from build123d import *

# Parameters (mm, degrees)
S2D0001_W           = 69.85
S2D0001_H           = 100.076
BOSS_EXTRUDE1_DEPTH = 3.175
FILLET1_R           = 3.175
S2D0002_R           = 1.27
CUT_EXTRUDE1_DEPTH  = 3.4925
BOSS_EXTRUDE2_DEPTH = 1.27
FILLET2_R           = 2.54
FILLET3_R           = 1.016
BOSS_EXTRUDE3_DEPTH = 6.35
S2D0005_W           = 5.08
S2D0005_H           = 6.35
BOSS_EXTRUDE4_DEPTH = 69.85
BOSS_EXTRUDE5_DEPTH = 0.889
BOSS_EXTRUDE6_DEPTH = 6.35


with BuildPart() as part:
    # S2D0001 → Boss-Extrude1 (new body)
    with BuildSketch(Plane(origin=(0, 0, 0), x_dir=(1, 0, 0), z_dir=(0, 1, 0))):
        with Locations((34.925, 50.038)):
            Rectangle(S2D0001_W, S2D0001_H)
    extrude(amount=-BOSS_EXTRUDE1_DEPTH)

    # Fillet1
    fillet1_edges = [part.edges().sort_by_distance(p)[0] for p in [
        (69.85, -1.5875, 0),
    ]]
    fillet(fillet1_edges, radius=FILLET1_R)

    # S2D0002 → Cut-Extrude1 (cut)
    with BuildSketch(Plane(origin=(0, 0, 0), x_dir=(1, 0, 0), z_dir=(0, 1, 0))):
        with Locations((3.175, 96.901)):
            Circle(S2D0002_R)
        with Locations((66.675, 96.901)):
            Circle(S2D0002_R)
        with Locations((3.175, 50.038)):
            Circle(S2D0002_R)
        with Locations((66.675, 50.038)):
            Circle(S2D0002_R)
        with Locations((3.175, 3.175)):
            Circle(S2D0002_R)
        with Locations((66.675, 3.175)):
            Circle(S2D0002_R)
    extrude(amount=-CUT_EXTRUDE1_DEPTH, mode=Mode.SUBTRACT)

    # Sketch3 → Boss-Extrude2 (add)
    with BuildSketch(Plane(origin=(0, 0, 0), x_dir=(-1, 0, 0), z_dir=(0, 1, 0))):
        with BuildLine():
            Line((-9.493170226, -96.266), (-59.69, -96.266))
            Line((-59.69, -96.266), (-66.04, -89.916))
            Line((-66.04, -89.916), (-66.04, -56.356170226))
            ThreePointArc((-66.04, -56.356170226), (-60.325, -50.038), (-66.04, -43.719829774))
            Line((-66.04, -43.719829774), (-66.04, -10.16))
            Line((-66.04, -10.16), (-59.69, -3.81))
            Line((-59.69, -3.81), (-16.51, -3.81))
            Line((-16.51, -3.81), (-3.81, -16.51))
            Line((-3.81, -16.51), (-3.81, -43.719829774))
            ThreePointArc((-3.81, -43.719829774), (-9.525, -50.038), (-3.81, -56.356170226))
            Line((-3.81, -56.356170226), (-3.81, -90.582829774))
            ThreePointArc((-3.81, -90.582829774), (-7.665128061, -92.410871939), (-9.493170226, -96.266))
        make_face()
    extrude(amount=BOSS_EXTRUDE2_DEPTH)

    # Fillet2
    fillet2_edges = [part.edges().sort_by_distance(p)[0] for p in [
        (3.81, 0.635, -16.51),
    ]]
    fillet(fillet2_edges, radius=FILLET2_R)

    # Fillet3
    fillet3_edges = [part.edges().sort_by_distance(p)[0] for p in [
        (38.1, 1.27, -3.81),
    ]]
    fillet(fillet3_edges, radius=FILLET3_R)

    # Sketch4 → Boss-Extrude3 (add)
    with BuildSketch(Plane.XZ.offset(3.175)):
        with BuildLine():
            Line((0, -96.901), (0, 0))
            Line((0, 0), (69.85, 0))
            Line((69.85, 0), (69.85, -96.901))
            ThreePointArc((69.85, -96.901), (68.92006403, -99.14606403), (66.675, -100.076))
            Line((66.675, -100.076), (3.175, -100.076))
            ThreePointArc((3.175, -100.076), (0.92993597, -99.14606403), (0, -96.901))
        make_face()
    extrude(amount=BOSS_EXTRUDE3_DEPTH)

    # S2D0005 → Boss-Extrude4 (add)
    with BuildSketch(Plane(origin=(0, 0, 0), x_dir=(0, 0, -1), z_dir=(1, 0, 0))):
        with Locations((12.7, -6.35)):
            Rectangle(S2D0005_W, S2D0005_H)
        with Locations((92.075, -6.35)):
            Rectangle(S2D0005_W, S2D0005_H)
    extrude(amount=BOSS_EXTRUDE4_DEPTH)

    # S2D0007 one side → Cut-Revolve1 (revolve, cut)
    with BuildSketch(Plane(origin=(12.7, -5.6261, -92.075), x_dir=(0, 1, 0), z_dir=(0, 0, 1))):
        Polygon((-2.7178, 0), (-1.3589, -0.816509495), (-1.3589, 12.7), (-2.7178, 12.7), align=None)
    revolve(axis=Axis((14.19233497, -6.985, -92.075), (-1, 0, 0)), mode=Mode.SUBTRACT)

    # Sketch7 one side → Cut-Revolve2 (revolve, cut)
    with BuildSketch(Plane(origin=(12.7, -5.6261, -12.7), x_dir=(0, 1, 0), z_dir=(0, 0, 1))):
        Polygon((-2.7178, 0), (-1.3589, -0.816509495), (-1.3589, 12.7), (-2.7178, 12.7), align=None)
    revolve(axis=Axis((14.19233497, -6.985, -12.7), (-1, 0, 0)), mode=Mode.SUBTRACT)

    # S2D0008 one side → Cut-Revolve3 (revolve, cut)
    with BuildSketch(Plane(origin=(57.15, -8.3439, -12.7), x_dir=(0, -1, 0), z_dir=(0, 0, 1))):
        Polygon((-2.7178, 0), (-1.3589, -0.816509495), (-1.3589, 12.7), (-2.7178, 12.7), align=None)
    revolve(axis=Axis((55.65766503, -6.985, -12.7), (1, 0, 0)), mode=Mode.SUBTRACT)

    # S2D0009 one side → Cut-Revolve4 (revolve, cut)
    with BuildSketch(Plane(origin=(57.15, -8.3439, -92.075), x_dir=(0, -1, 0), z_dir=(0, 0, 1))):
        Polygon((-2.7178, 0), (-1.3589, -0.816509495), (-1.3589, 12.7), (-2.7178, 12.7), align=None)
    revolve(axis=Axis((55.65766503, -6.985, -92.075), (1, 0, 0)), mode=Mode.SUBTRACT)

    # Sketch10 → Boss-Extrude5 (add)
    with BuildSketch(Plane.XZ.offset(9.525)):
        with BuildLine():
            Line((0, -94.615), (0, -89.535))
            Line((0, -89.535), (6.35, -89.535))
            ThreePointArc((6.35, -89.535), (8.89, -92.075), (6.35, -94.615))
            Line((6.35, -94.615), (0, -94.615))
        make_face()
        with BuildLine():
            Line((0, -15.24), (0, -10.16))
            Line((0, -10.16), (6.35, -10.16))
            ThreePointArc((6.35, -10.16), (8.89, -12.7), (6.35, -15.24))
            Line((6.35, -15.24), (0, -15.24))
        make_face()
        with BuildLine():
            Line((69.85, -10.16), (69.85, -15.24))
            Line((69.85, -15.24), (63.5, -15.24))
            ThreePointArc((63.5, -15.24), (60.96, -12.7), (63.5, -10.16))
            Line((63.5, -10.16), (69.85, -10.16))
        make_face()
        with BuildLine():
            Line((69.85, -89.535), (69.85, -94.615))
            Line((69.85, -94.615), (63.5, -94.615))
            ThreePointArc((63.5, -94.615), (60.96, -92.075), (63.5, -89.535))
            Line((63.5, -89.535), (69.85, -89.535))
        make_face()
    extrude(amount=BOSS_EXTRUDE5_DEPTH)

    # S2D0019 one side → Cut-Revolve5 (revolve, cut)
    with BuildSketch(Plane(origin=(4.9911, -4.064, -92.075), x_dir=(-1, 0, 0), z_dir=(0, 0, 1))):
        Polygon((-2.7178, 0), (-1.3589, -0.816509495), (-1.3589, 6.35), (-2.7178, 6.35), align=None)
    revolve(axis=Axis((6.35, -2.88916503, -92.075), (0, -1, 0)), mode=Mode.SUBTRACT)

    # Sketch12 one side → Cut-Revolve6 (revolve, cut)
    with BuildSketch(Plane(origin=(62.1411, -4.064, -92.075), x_dir=(-1, 0, 0), z_dir=(0, 0, 1))):
        Polygon((-2.7178, 0), (-1.3589, -0.816509495), (-1.3589, 6.35), (-2.7178, 6.35), align=None)
    revolve(axis=Axis((63.5, -2.88916503, -92.075), (0, -1, 0)), mode=Mode.SUBTRACT)

    # S2D0021 one side → Cut-Revolve7 (revolve, cut)
    with BuildSketch(Plane(origin=(62.1411, -4.064, -12.7), x_dir=(-1, 0, 0), z_dir=(0, 0, 1))):
        Polygon((-2.7178, 0), (-1.3589, -0.816509495), (-1.3589, 6.35), (-2.7178, 6.35), align=None)
    revolve(axis=Axis((63.5, -2.88916503, -12.7), (0, -1, 0)), mode=Mode.SUBTRACT)

    # Sketch14 one side → Cut-Revolve8 (revolve, cut)
    with BuildSketch(Plane(origin=(4.9911, -4.064, -12.7), x_dir=(-1, 0, 0), z_dir=(0, 0, 1))):
        Polygon((-2.7178, 0), (-1.3589, -0.816509495), (-1.3589, 6.35), (-2.7178, 6.35), align=None)
    revolve(axis=Axis((6.35, -2.88916503, -12.7), (0, -1, 0)), mode=Mode.SUBTRACT)

    # Sketch15 → Boss-Extrude6 (add)
    with BuildSketch(Plane.XZ.offset(9.525)):
        Polygon((69.683605301, 0), (65.111605301, 8.4836), (60.895205301, 8.4836), (60.895205301, 2.8194), (12.9794, 2.8194), (12.9794, 8.4836), (0, 8.4836), (0, 0), align=None)
    extrude(amount=-BOSS_EXTRUDE6_DEPTH)


solid = part.part
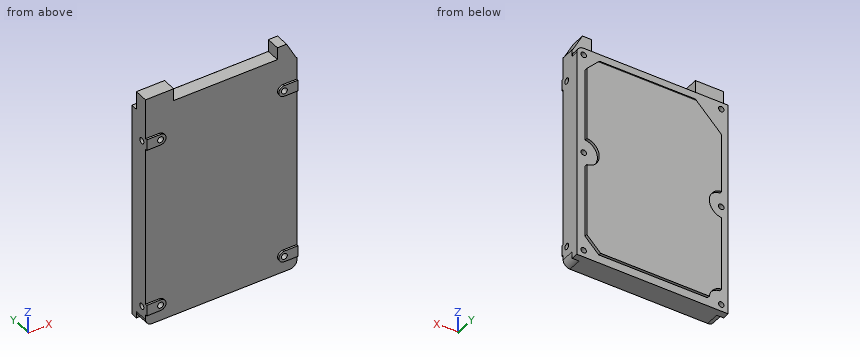
Verification items for the finished model (mm, model axes). Coordinates: 2 decimals unless noted, no trailing zeros. Write each loop counter-clockwise with the first axis right and the second up, starting at its lowest first coordinate (ties: lowest second). Pieces come first, ordered by that corner, then holes. Notation, with made-up numbers: M 49.5,-4.75 L 90.5,-4.75 A9 cw 90.5,5.25 Z; hole C 56.25,35.5 d7. An arc over 180 degrees is marked long. Use a Markdown table: item, result.
Q1. Go/stop test with flat-tipped pins: P1, Ø12, axis at x = 20, z = -13.5, coming from the -Y side (3 decimals); P2, Ø6, axis at x = 56.5, y = -7, coming from the +Z side; P3, Ø1.3, axis at x = 66.5, z = -3.5, coming from the +Y side (3 decimals). Record where each tip stops, or that it passes through.
Reply:
| item | result |
|---|---|
| P1 | stops at y = -9.525 |
| P2 | stops at z = 2.82 |
| P3 | stops at y = -3.175 |
Q2. Sectioned sample at A-A, the plane x = 32.5. Record the boundary of the cut face in (y, z) (3 decimals), plus the area to 3 significant figures.
Reply:
| item | result |
|---|---|
| outline | M -9.525,-100.076 L 0,-100.076 L 0,-96.266 L 1.27,-96.266 L 1.27,-4.826 A1.016 ccw 0.254,-3.81 L 0,-3.81 L 0,0 L -3.175,0 L -3.175,2.819 L -9.525,2.819 Z |
| area | 1,090 mm² |
Q3. Sectioned sample at C-C, the plane y = -2. Record the boundary of the cut face in (x, z) (3 decimals).
Reply:
| item | result |
|---|---|
| outline | M 0,-100.076 L 69.85,-100.076 L 69.85,-3.175 A3.175 ccw 66.675,0 L 0,0 Z; hole C 3.175,-96.901 d2.54; hole C 3.175,-50.038 d2.54; hole C 3.175,-3.175 d2.54; hole C 66.675,-96.901 d2.54; hole C 66.675,-50.038 d2.54; hole C 66.675,-3.175 d2.54 |
Q4. Thickness scan on line 1 (X direction, y = -8.9, z = -12.7); line 2 (Z direction, x = 66.5, y = -2.25); line 3 (Z direction, x = 6.35, y = -5.7). Record the ranges inside material, lowest first.
Reply:
| item | result |
|---|---|
| line 1 | x = 0 to 4.99, 7.71 to 62.14, 64.86 to 69.85 |
| line 2 | z = -100.08 to -98.16, -95.64 to -51.3, -48.78 to -4.43, -1.92 to 0 |
| line 3 | z = -100.08 to -93.43, -90.72 to -14.06, -11.34 to 8.48 |
Q5. Sectioned sample at D-D, the plane z = -79.5. Record the boundary of the cut face in (x, y) (3 decimals).
Reply:
| item | result |
|---|---|
| outline | M 0,-9.525 L 69.85,-9.525 L 69.85,0 L 66.04,0 L 66.04,1.27 L 3.81,1.27 L 3.81,0 L 0,0 Z |
Q6. Sectioned sample at B-B, the plane z = -6.5. Record the boundary of the cut face in (x, y) (3 decimals).
Reply:
| item | result |
|---|---|
| outline | M 0,-9.525 L 69.85,-9.525 L 69.85,0 L 62.38,0 L 62.38,1.27 L 13.82,1.27 L 13.82,0 L 0,0 Z |
